For this review, take the finished solid that the model builds, in its own axes (mm). Face numbers are marked on the shaded views. Round coordinates to 2 decimals unless told otherwise and drop trailing zeros. Loops run counter-clockwise (first coordinate to the right, second up) from the corner with the lowest first, then second, coordinate; pieces in that order, holes last. Notation, with made-up numbers: (32, 30.5) -> (75, 30.5) arc R31 ccw to (75, 61.5) -> close; hole circle Ø7 at (67, -8). An arc over 180 degrees is marked (long way). Write each question's results on one line, items separated by ' | '.
```python
from build123d import *

# Parameters (mm, degrees)
F1_DEPTH      = 332.5
F1_DEPTH_BACK = 332.5
F2_R          = 4.99999
F3_W          = 65
F3_H          = 175
F4_DEPTH      = 5
F5_R          = 2
F7_D          = 13


# Not quite as in the source:
# - a fillet or chamfer is up to 0.001 mm smaller than in the source, because OpenCascade refuses the exact size
# - a pattern or mirror of a feature is missing from the dataset's text; its kind, count and spacing are read off the source's solid
# - a feature names something its author has since deleted; it is built from what else it names


with BuildPart() as f1:
    # F0 (on Front) → F1 (new body, two sides)
    with BuildSketch(Plane.XZ) as f1_sk:
        Polygon((0, 28.2842712475), (-28.2842712475, 0), (-24.7487373415, -3.5355339059), (0, 21.2132034356), (24.7487373415, -3.5355339059), (28.2842712475, 0), align=None)
    extrude(amount=F1_DEPTH)
    extrude(f1_sk.sketch, amount=-F1_DEPTH_BACK)

    # F2 (radius 5 in the source; OpenCascade refuses exactly that, so slightly less here)
    f2_edges = [f1.edges().sort_by_distance(p)[0] for p in [
        (24.748737, 0, -3.535534),
        (0, 0, 21.213203),
        (-24.748737, 0, -3.535534),
    ]]
    fillet(f2_edges, radius=F2_R)

    # F3 (on face) → F4 (join)
    with BuildSketch(Plane.XZ.offset(332.5)):
        with Locations((0, 86.0355339059)):
            Rectangle(F3_W, F3_H)
    f4 = extrude(amount=F4_DEPTH)

    # F4_copies: F4 across plane
    add(f4.mirror(Plane.ZX))

    # F5
    f5_edges = [f1.edges().sort_by_distance(p)[0] for p in [
        (32.5, -335, 173.535534),
        (32.5, -335, -1.464466),
        (-32.5, -335, 173.535534),
        (-32.5, -335, -1.464466),
        (-32.5, 335, -1.464466),
        (32.5, 335, -1.464466),
        (-32.5, 335, 173.535534),
        (32.5, 335, 173.535534),
    ]]
    fillet(f5_edges, radius=F5_R)

    # F7 (through all)
    with Locations(Plane.XZ.offset(337.5)):
        with Locations((0, 63.5355339059), (0, 133.5355339059)):
            Hole(F7_D / 2)


solid = f1.part
```
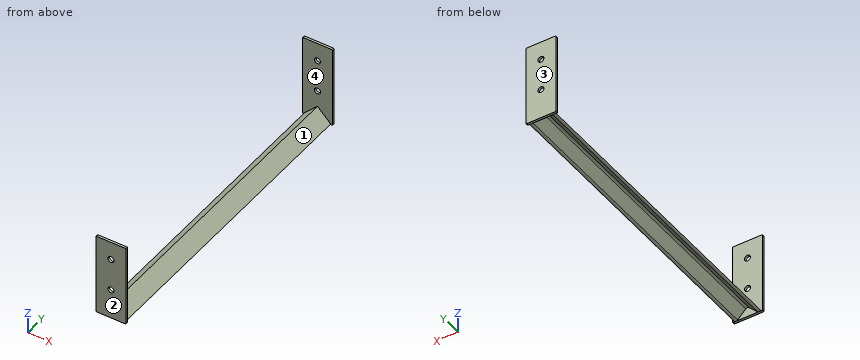
1. To check wall thickness, follow probe 1 along Z at (x, y) = (0, 333.8); probe 2 along Y at (x, z) = (1.5, 102.5); probe 3 along Z at (x, y) = (15, 19). State the ranges of each line that lie inside material, in increasing order.
Values found:
probe 1: z = -1.46 to 57.04, 70.04 to 127.04, 140.04 to 173.54 | probe 2: y = -337.5 to -332.5, 332.5 to 337.5 | probe 3: z = 6.21 to 13.28
2. For pin 1 (8 mm diameter, centred on x = -3.5, y = 54, fed in from +Z); pin 2 (21 mm diameter, centred on x = 0, z = 133.54, fed in from +Y); pin 3 (10 mm diameter, centred on x = -12.5, y = -258.5, fed in from -Z); pin 4 (5 mm diameter, centred on x = -13.5, y = -8.5, fed in from +Z), all flat-tipped, find the tip position at first contact; note any pin that passes through.
Values found:
pin 1: stops at z = 28.28 | pin 2: stops at y = 337.5 | pin 3: stops at z = 3.71 | pin 4: stops at z = 17.28
3. Consider section A-A (z = 115). State the section outline as (x, y) points.
Values found:
outline: (-32.5, -337.5) -> (32.5, -337.5) -> (32.5, -332.5) -> (-32.5, -332.5) -> close; (-32.5, 332.5) -> (32.5, 332.5) -> (32.5, 337.5) -> (-32.5, 337.5) -> close
4. Consider section C-C (z = 11). State the section outline as (x, y) points.
Values found:
outline: (-32.5, -337.5) -> (32.5, -337.5) -> (32.5, -332.5) -> (17.28, -332.5) -> (17.28, 332.5) -> (32.5, 332.5) -> (32.5, 337.5) -> (-32.5, 337.5) -> (-32.5, 332.5) -> (-17.28, 332.5) -> (-17.28, -332.5) -> (-32.5, -332.5) -> close; hole (-10.21, -332.5) -> (10.21, -332.5) -> (10.21, 332.5) -> (-10.21, 332.5) -> close
5. Draft analysis for pull direction Y (two halves, no side actions). For the marked faces 1, 2, 3 and 4, state which applies: released by +Y, released by -Y, zero draft, split by the parting line, or undercut.
Values found:
face 1: undercut | face 2: released by -Y | face 3: released by +Y | face 4: undercut
